Autodesk Inventor part; units mm, degrees
ref_plane "Work Plane2" through (0, 13, -25.5) normal (-1, 0, 0) x (0, 0, 1)
ref_plane "YZ Plane" through (0, 0, 0) normal (1, 0, 0) x (0, 1, 0)
ref_plane "XZ Plane" through (0, 0, 0) normal (0, 1, 0) x (-1, 0, 0)
sketch "Sketch1" plane through (0, 0, 0) normal (0, 1, 0) x (-1, 0, 0)
  line L0 (37.5, 30) -> (-37.5, 30)
  line L1 (-37.5, 30) -> (-37.5, -30)
  line L2 (-37.5, -30) -> (37.5, -30)
  line L3 (37.5, -30) -> (37.5, 30)
  line L4 (37.5, 30) -> (-37.5, -30) construction
  line L5 (-37.5, 30) -> (37.5, -30) construction
  line L6 (38, 30.5) -> (-38, 30.5)
  line L7 (-38, 30.5) -> (-38, -30.5)
  line L8 (-38, -30.5) -> (38, -30.5)
  line L9 (38, -30.5) -> (38, 30.5)
  line L10 (38, 30.5) -> (-38, -30.5) construction
  line L11 (-38, 30.5) -> (38, -30.5) construction
  point P0 (0, 0)
  dimension "d0" = 75
  dimension "d1" = 60
  dimension "d2" = 76
  dimension "d3" = 61
extrude "Extrusion1" add sketch "Sketch1" along normal blind 35
sketch "Sketch2" plane through (0, 0, 0) normal (0, -1, 0) x (1, 0, 0)
  line L0 (37.5, -30) -> (37.5, 30)
  line L1 (-37.5, 30) -> (37.5, 30)
  line L2 (37.5, 30) -> (37.5, -30)
  line L3 (37.5, -30) -> (-37.5, -30)
  line L4 (-37.5, -30) -> (-37.5, 30)
  line L5 (-37.5, 30) -> (37.5, -30) construction
  line L6 (37.5, 30) -> (-37.5, -30) construction
  point P0 (0, 0)
extrude "Extrusion2" add sketch "Sketch2" against normal blind 0.5
sketch "Sketch4" plane through (-38, 0, -30.5) normal (-1, 0, 0) x (0, 0, 1)
  line L0 (61, 35) -> (0, 35)
  line L1 (0, 35) -> (5, 35)
  line L2 (61, 35) -> (56, 35)
  line L3 (30.5, 0) -> (30.5, 8)
  line L4 (5, 35) -> (56, 35)
  line L5 (56, 35) -> (56, 13)
  line L6 (56, 13) -> (5, 13)
  line L7 (5, 13) -> (5, 35)
  line L8 (5, 35) -> (56, 35)
  line L9 (56, 35) -> (56, 8)
  line L10 (56, 8) -> (5, 8)
  line L11 (5, 8) -> (5, 35)
  point P0 (5, 13)
  dimension "d8" = 5
  dimension "d9" = 5
  dimension "d10" = 8
extrude "Extrusion3" cut sketch "Sketch4" against normal blind 30
sketch "Sketch6" plane through (38, 0, -30.5) normal (0, 0, -1) x (-1, 0, 0)
  line L0 (0, 0) -> (0, 35)
  line L1 (0, 0) -> (76, 0)
  line L2 (0, 35) -> (76, 35)
  line L3 (76, 35) -> (76, 0)
  line L4 (76, 0) -> (0, 0)
  line L5 (0, 0) -> (0, 35)
  point P0 (38, 0)
extrude "Extrusion4" add sketch "Sketch6" along normal blind 2
sketch "Sketch7" plane through (-38, 0, 30.5) normal (0, 0, 1) x (1, 0, 0)
  line L0 (76, 0) -> (76, 35)
  line L1 (0, 0) -> (0, 35)
  line L2 (76, 35) -> (0, 35)
  line L3 (0, 35) -> (0, 0)
  line L4 (0, 0) -> (76, 0)
  line L5 (76, 0) -> (76, 35)
  point P0 (38, 0)
  point P1 (0, 35)
extrude "Extrusion5" add sketch "Sketch7" along normal blind 2
sketch "Sketch8" plane through (-38, 13, -25.5) normal (-1, 0, 0) x (0, 0, 1)
  line L0 (0, 22) -> (-7, 22)
  line L1 (58, -13) -> (-7, -13)
  line L2 (-7, 22) -> (58, 22)
  line L3 (58, 22) -> (58, -13)
  line L4 (58, -13) -> (-7, -13)
  line L5 (-7, -13) -> (-7, 22)
  point P0 (25.5, -13)
  point P1 (0, 22)
  point P2 (-7, -13)
extrude "Extrusion6" add sketch "Sketch8" along normal blind 2
sketch "Sketch10" plane through (38, 0, -32.5) normal (1, 0, 0) x (0, 0, -1)
  line L0 (-65, 35) -> (0, 35)
  line L1 (0, 0) -> (-65, 0)
  line L2 (0, 35) -> (-65, 35)
  line L3 (-65, 35) -> (-65, 0)
  line L4 (-65, 0) -> (0, 0)
  line L5 (0, 0) -> (0, 35)
  point P0 (-32.5, 0)
  point P1 (-7, 35)
  point P2 (-7, 35)
extrude "Extrusion8" add sketch "Sketch10" along normal blind 2
sketch "Sketch12" plane through (-40, 13, -25.5) normal (-1, 0, 0) x (0, 0, 1)
  line L0 (0, 22) -> (0, -5)
  line L1 (0, -5) -> (51, -5)
  line L2 (0, 22) -> (51, 22)
  line L3 (51, 22) -> (51, -5)
  line L4 (51, -5) -> (0, -5)
  line L5 (0, -5) -> (0, 22)
  point P0 (25.5, -13)
extrude "Extrusion9" cut sketch "Sketch12" against normal blind 30
ref_plane "Work Plane2" through (0, 13, -25.5) normal (-1, 0, 0) x (0, 0, 1)
mirror "Mirror3" about plane through (0, 13, -25.5) normal (-1, 0, 0) of "Extrusion3", "Extrusion9"
sketch "Sketch13" plane through (-40, 13, -25.5) normal (-1, 0, 0) x (0, 0, 1)
  line L0 (0, 22) -> (0, -5)
  line L1 (0, 22) -> (0, 18)
  line L2 (51, -5) -> (51, 22)
  line L3 (51, 22) -> (51, 18)
  line L4 (-7, 22) -> (-7, -13)
  line L5 (-7, 18) -> (-5.5, 18)
  line L6 (-7, 18) -> (-5.5, 18) construction
  line L7 (51, 22) -> (51, 18)
  line L8 (58, -13) -> (58, 22)
  line L9 (58, 18) -> (56.5, 18)
  line L10 (-5.5, 18) -> (56.5, 18)
  line L11 (56.5, 18) -> (56.5, 19)
  line L12 (56.5, 19) -> (-5.5, 19)
  line L13 (-5.5, 19) -> (-5.5, 18)
  point P0 (25.5, -13)
  dimension "d25" = 4
  dimension "d26" = 1.5
  dimension "d27" = 0
  dimension "d28" = 4
  dimension "d29" = 1.5
  dimension "d30" = 1
extrude "Extrusion10" cut sketch "Sketch13" against normal blind 78.5
properties part number "3 Pzem test"
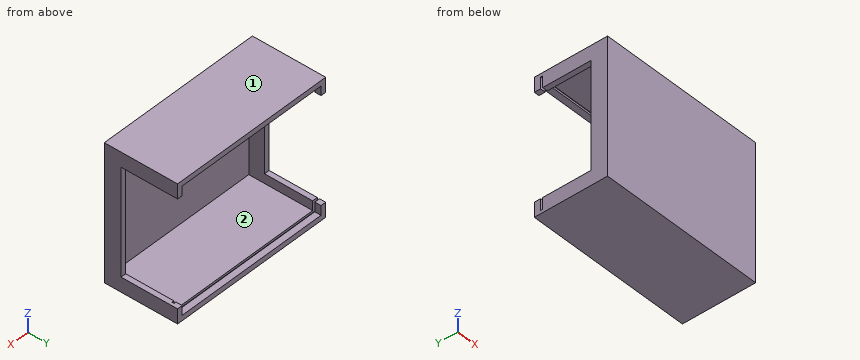
CAD build for the part. Positions are in the model's coordinates, mm. Face numbers are marked on the shaded views. A direction names the side the tool comes from. Round coordinates to 2 decimals unless told otherwise and drop trailing zeros. Write each loop counter-clockwise with the first axis right and the second up, starting at its lowest first coordinate (ties: lowest second). Pieces come first, ordered by that corner, then holes.
(1) Slice it at A-A, the plane y = 16.5. Write the cut outline in (x, z).
(2) Slice it at D-D, the plane x = -31. Write the cut outline in (y, z), and give its area (3 significant figures).
(3) Drop flat-ended pins along their axis: P1, Ø2, axis at x = 39, z = 1.5, coming from the +Y side; P2, Ø6, axis at x = -5, z = 16, coming from the +Y side; P3, Ø0.5, axis at y = 31.5, z = -29.5, coming from the -X side. Give the stop position or say it passes through.
(4) Slice it at C-C, the plane y = 4. Write the cut outline in (x, z), and give its area (3 significant figures).
(5) Slice it at B-B, the plane z = 21. Write the cut outline in (x, y), and give its area (3 significant figures).
(6) 3-axis set-ups, long thin cutter, end or side, ignore diameter. For the marked faces 1 and 2: which of +Z, -Z, +X, -X, +Y, -Y reach the whole face in a straight line?
(7) Probe line 1 along Z through (x, y) = (-5, 25.5); line 2 along X through (y, z) = (3, 0.5); line 3 along Y through (x, z) = (-34, -23). List the from-to ranges inside material, lowest first.
From the geometry:
1. outline: (-40, -32.5) - (40, -32.5) - (40, -25.5) - (37.5, -25.5) - (37.5, -30) - (-37.5, -30) - (-37.5, -25.5) - (-40, -25.5) - close; (-40, 25.5) - (-37.5, 25.5) - (-37.5, 30) - (37.5, 30) - (37.5, 25.5) - (40, 25.5) - (40, 32.5) - (-40, 32.5) - close
2. outline: (0, -32.5) - (35, -32.5) - (35, -30) - (32, -30) - (32, -31) - (31, -31) - (31, -30) - (0.5, -30) - (0.5, 30) - (31, 30) - (31, 31) - (32, 31) - (32, 30) - (35, 30) - (35, 32.5) - (0, 32.5) - close
2. area: 203 mm2
3. P1: stops at y = 8
3. P2: stops at y = 0.5
3. P3: stops at x = 38.5
4. outline: (-40, -32.5) - (40, -32.5) - (40, 32.5) - (-40, 32.5) - close; hole (-37.5, -30) - (37.5, -30) - (37.5, 30) - (-37.5, 30) - close
4. area: 700 mm2
5. outline: (-40, 0) - (40, 0) - (40, 8) - (37.5, 8) - (37.5, 0.5) - (-37.5, 0.5) - (-37.5, 8) - (-40, 8) - close
5. area: 77.5 mm2
6. face 1: +Z, +X, -X, +Y, -Y
6. face 2: +Y
7. line 1: z = -32.5 to -30, 30 to 32.5
7. line 2: x = -40 to -37.5, 37.5 to 40
7. line 3: y = 0 to 0.5
